Read the model definition and answer for the solid it produces. Units are mm, in the model's axes. A direction names the side the tool comes from. Round coordinates to 2 decimals unless told otherwise and drop trailing zeros. Loops run counter-clockwise (first coordinate to the right, second up) from the corner with the lowest first, then second, coordinate; pieces in that order, holes last. Notation, with made-up numbers: (12, 50) - (70, 50) arc R16 ccw to (70, 81) - close; hole circle Ø5 at (-1.75, -34.75). An arc over 180 degrees is marked (long way). Use one line per item in the form item = value. Start each with the question number.
```python
from build123d import *

# Parameters (mm, degrees)
SKETCH_1_W          = 15
SKETCH_1_H          = 15
EXTRUDE_1_DEPTH     = 9.5
CUT_EXTRUDE_1_DEPTH = 7
SKETCH_5_R          = 0.75
EXTRUDE_2_DEPTH     = 1.5
CUT_EXTRUDE_2_REACH = 17.281
SKETCH_6_R          = 3


with BuildPart() as part:
    # 草图1 → 凸台-拉伸1 (new body)
    with BuildSketch(Plane(origin=(0, 0, 0), x_dir=(1, 0, 0), z_dir=(0, 1, 0))):
        Rectangle(SKETCH_1_W, SKETCH_1_H)
    extrude(amount=EXTRUDE_1_DEPTH)

    # 草图2 → 切除-拉伸1 (cut)
    with BuildSketch(Plane(origin=(0, 9.5, 0), x_dir=(-1, 0, 0), z_dir=(0, 1, 0))):
        with BuildLine():
            Line((6.5, -5.5), (7, -5.5))
            Line((7, -5.5), (7, 5.5))
            Line((7, 5.5), (6.5, 5.5))
            ThreePointArc((6.5, 5.5), (5.792893219, 5.792893219), (5.5, 6.5))
            Line((5.5, 6.5), (5.5, 7))
            Line((5.5, 7), (-5.5, 7))
            Line((-5.5, 7), (-5.5, 6.5))
            ThreePointArc((-5.5, 6.5), (-5.792893219, 5.792893219), (-6.5, 5.5))
            Line((-6.5, 5.5), (-7, 5.5))
            Line((-7, 5.5), (-7, -5.5))
            Line((-7, -5.5), (-6.5, -5.5))
            ThreePointArc((-6.5, -5.5), (-5.792893219, -5.792893219), (-5.5, -6.5))
            Line((-5.5, -6.5), (-5.5, -7))
            Line((-5.5, -7), (5.5, -7))
            Line((5.5, -7), (5.5, -6.5))
            ThreePointArc((5.5, -6.5), (5.792893219, -5.792893219), (6.5, -5.5))
        make_face()
    extrude(amount=-CUT_EXTRUDE_1_DEPTH, mode=Mode.SUBTRACT)

    # 草图5 → 凸台-拉伸2 (add)
    with BuildSketch(Plane(origin=(0, 9.5, 0), x_dir=(-1, 0, 0), z_dir=(0, 1, 0))):
        with Locations(Location((6.5, -6.5, 0), (0, 0, 270))):
            Circle(SKETCH_5_R)
        with Locations(Location((6.5, 6.5, 0), (0, 0, 270))):
            Circle(SKETCH_5_R)
        with Locations(Location((-6.5, 6.5, 0), (0, 0, 270))):
            Circle(SKETCH_5_R)
        with Locations(Location((-6.5, -6.5, 0), (0, 0, 270))):
            Circle(SKETCH_5_R)
    extrude(amount=EXTRUDE_2_DEPTH)

    # 草图6 → 切除-拉伸2 (cut, up to next)
    with BuildSketch(Plane.XZ, mode=Mode.PRIVATE) as cut_extrude_2_sk1:
        with Locations(Location((0, 0, 0), (0, 0, 270))):
            Circle(SKETCH_6_R)
    cut_extrude_2_tool1 = extrude(cut_extrude_2_sk1.sketch, amount=-CUT_EXTRUDE_2_REACH, mode=Mode.PRIVATE) & part.part
    add(cut_extrude_2_tool1.solids().sort_by_distance((0, 0, 0))[0], mode=Mode.SUBTRACT)


solid = part.part
```
1) Determine the mould class of faces 1 (the cylindrical face through (5.801, 6.049, -5.785)), 2 (the flat face through (0, 5, -7.5)), 3 (the cylindrical face through (-5.785, 6.049, -5.801)), 4 (the flat face through (6.5, 11, 6.5)) for opening direction Z: +Z half, -Z half, draft (parallel to the pull), parting line (faces both ways), or undercut.
2) Straight lines are drawn through the part: line 1 (X direction, y = 1.5, z = 0); line 2 (X direction, y = 9.25, z = 5). For each, find the intervals that lie inside material, in ascending order. Write a range as from..to.
3) A cutting plane is placed at A-A on x = 0. Write down the section's boundary in (y, z), plus the area to 3 significant figures.
4) For faces 5 (the flat face through (-7, 6, 0)), 6 (the cylindrical face through (0.9, 1.23, -2.86)), determine the directions among +Z, -Z, +X, -X, +Y, -Y from which every point of the face is accessible in a straight line to the end or side of a thin tool.
5) A cutting plane is placed at D-D on y = 9.75. Write down the section's boundary in (x, z).
6) A cutting plane is placed at B-B on z = 0. Write down the section's boundary in (x, y).
7) A cutting plane is placed at C-C on y = 2. Write down the section's boundary in (x, z), plus the area to 3 significant figures.
8) A flat-ended cylindrical pin translates along its axis: pin 1 (8 mm diameter, centred on x = 0, z = 0, fed in from +Y). Find the tip coordinate at first contact, or state that the pin passes through.
Checks:
q1.face_1 = undercut
q1.face_2 = -Z half
q1.face_3 = undercut
q1.face_4 = draft
q2.line_1 = -7.5..-3, 3..7.5
q2.line_2 = -7.5..-7, 7..7.5
q3.outline = (0, -7.5) - (9.5, -7.5) - (9.5, -7) - (2.5, -7) - (2.5, -3) - (0, -3) - close; (0, 3) - (2.5, 3) - (2.5, 7) - (9.5, 7) - (9.5, 7.5) - (0, 7.5) - close
q3.area = 29.5 mm²
q4.face_5 = +Y
q4.face_6 = +Y, -Y
q5.outline = circle Ø1.5 at (-6.5, -6.5); circle Ø1.5 at (-6.5, 6.5); circle Ø1.5 at (6.5, -6.5); circle Ø1.5 at (6.5, 6.5)
q6.outline = (-7.5, 0) - (-3, 0) - (-3, 2.5) - (-7, 2.5) - (-7, 9.5) - (-7.5, 9.5) - close; (3, 0) - (7.5, 0) - (7.5, 9.5) - (7, 9.5) - (7, 2.5) - (3, 2.5) - close
q7.outline = (-7.5, -7.5) - (7.5, -7.5) - (7.5, 7.5) - (-7.5, 7.5) - close; hole circle Ø6 at (0, 0)
q7.area = 197 mm²
q8.pin_1 = 2.5
